Verification items for the finished model (mm, model axes). A direction names the side the tool comes from. Coordinates: 2 decimals unless noted, no trailing zeros. Write each loop counter-clockwise with the first axis right and the second up, starting at its lowest first coordinate (ties: lowest second). Pieces come first, ordered by that corner, then holes. Notation, with made-up numbers: (73.5, -12.75) -> (111.5, -12.75) arc R19 cw to (111.5, -6.75) -> close; hole circle Ø4 at (76, 29.5). An arc over 180 degrees is marked (long way). Answer in a Markdown table with one row per item.
```python
from build123d import *

# Parameters (mm, degrees)
SKETCH1_W           = 88.5
SKETCH1_H           = 78
SKETCH1_W_2         = 10
SKETCH1_H_2         = 58
BOSS_EXTRUDE1_DEPTH = 10
M4_TAPPED_HOLE1_D   = 3.3


with BuildPart() as part:
    # Sketch1 → Boss-Extrude1 (new body)
    with BuildSketch(Plane(origin=(0, 0, 0), x_dir=(0, 0, -1), z_dir=(1, 0, 0))):
        Rectangle(SKETCH1_W, SKETCH1_H)
        with Locations((-19.25, 0)):
            Rectangle(SKETCH1_W_2, SKETCH1_H_2, mode=Mode.SUBTRACT)
        with Locations((29.25, 0)):
            Rectangle(SKETCH1_W_2, SKETCH1_H_2, mode=Mode.SUBTRACT)
    extrude(amount=BOSS_EXTRUDE1_DEPTH)

    # M4 Tapped Hole1 (through all)
    with Locations(Plane(origin=(10, 0, 0), x_dir=(0, 0, -1), z_dir=(1, 0, 0))):
        with Locations((-2.25, -30.75), (-2.25, 30.75), (2.25, -30.75), (2.25, 30.75)):
            Hole(M4_TAPPED_HOLE1_D / 2)


solid = part.part
```
1. Release check for a two-part mould opening along Z. For faces 3 (the face through (5, 39, 1)), 4 (the face through (5, 29, 19)), 5 (the face through (5, -1, -44.25)) record: released by +Z, released by -Z, zero draft, split by the parting line, or undercut.
Findings below:
| item | result |
|---|---|
| face 3 | zero draft |
| face 4 | undercut |
| face 5 | released by -Z |
2. Sectioned sample at D-D, the plane z = 2.25. Record the cut outline in (x, y).
Findings below:
| item | result |
|---|---|
| outline | (0, -39) -> (10, -39) -> (10, -32.4) -> (0, -32.4) -> close; (0, -29.1) -> (10, -29.1) -> (10, 29.1) -> (0, 29.1) -> close; (0, 32.4) -> (10, 32.4) -> (10, 39) -> (0, 39) -> close |
3. Sectioned sample at B-B, the plane y = -30.75. Record the cut outline in (x, z), and give its area (3 significant figures).
Findings below:
| item | result |
|---|---|
| outline | (0, -44.25) -> (10, -44.25) -> (10, -3.9) -> (0, -3.9) -> close; (0, -0.6) -> (10, -0.6) -> (10, 0.6) -> (0, 0.6) -> close; (0, 3.9) -> (10, 3.9) -> (10, 44.25) -> (0, 44.25) -> close |
| area | 819 mm² |
4. Sectioned sample at C-C, the plane x = 6. Record the cut outline in (y, z), and give its area (3 significant figures).
Findings below:
| item | result |
|---|---|
| outline | (-39, -44.25) -> (39, -44.25) -> (39, 44.25) -> (-39, 44.25) -> close; hole circle Ø3.3 at (-30.75, -2.25); hole circle Ø3.3 at (-30.75, 2.25); hole (-29, -34.25) -> (29, -34.25) -> (29, -24.25) -> (-29, -24.25) -> close; hole (-29, 14.25) -> (29, 14.25) -> (29, 24.25) -> (-29, 24.25) -> close; hole circle Ø3.3 at (30.75, -2.25); hole circle Ø3.3 at (30.75, 2.25) |
| area | 5,710 mm² |
5. Material ranges on probe 1 along Y at (x, z) = (8, 2.25); probe 2 along Z at (x, y) = (7.5, -23.5); probe 3 along Y at (x, z) = (7, -30), recorded low to high. Write a range as from..to.
Findings below:
| item | result |
|---|---|
| probe 1 | y = -39..-32.4, -29.1..29.1, 32.4..39 |
| probe 2 | z = -44.25..-34.25, -24.25..14.25, 24.25..44.25 |
| probe 3 | y = -39..-29, 29..39 |
6. Access from +Z, -Z, +X, -X, +Y, -Y to the whole of each face (thin tool, end or side, straight path). Record for faces 1 (the face through (5, 0, 24.25)), 2 (the face through (0, 1, 1)).
Findings below:
| item | result |
|---|---|
| face 1 | +X, -X |
| face 2 | +Z, -Z, -X, +Y, -Y |
7. Sectioned sample at A-A, the plane z = -28. Record the cut outline in (x, y), and give its area (3 significant figures).
Findings below:
| item | result |
|---|---|
| outline | (0, -39) -> (10, -39) -> (10, -29) -> (0, -29) -> close; (0, 29) -> (10, 29) -> (10, 39) -> (0, 39) -> close |
| area | 200 mm² |
8. Go/stop test with a flat-tipped pin: pin 1 (4 mm diameter, centred on y = 30.75, z = -2.25, fed in from +X). Record where the tip stops, or that it passes through.
Findings below:
| item | result |
|---|---|
| pin 1 | stops at x = 10 |
